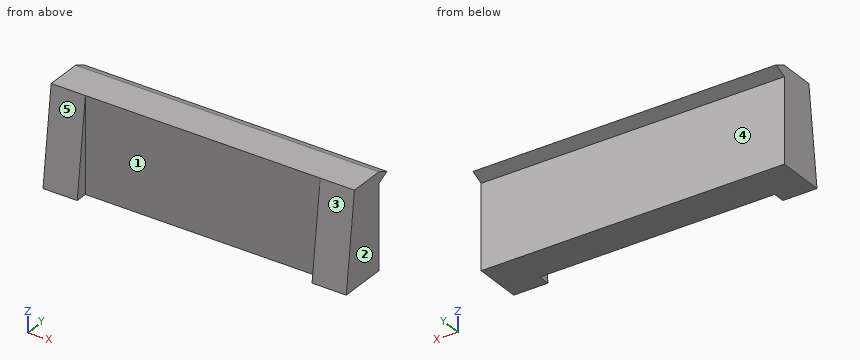
from build123d import *

# Parameters (mm, degrees)
F1_DEPTH = 12.75
F2_W     = 9.87
F2_H     = 0.5
F3_DEPTH = 4.001


with BuildPart() as f1:
    # F0 (on Right) → F1 (new body)
    with BuildSketch(Plane.YZ):
        Polygon((1.5, 4), (0, 4), (-0.5, 0), (1.5, 0), (1.5, 3.533692), (2, 3.766846), align=None)
    extrude(amount=F1_DEPTH)

    # F2 (on face) → F3 (cut, through all)
    with BuildSketch(Plane(origin=(0, 0, 0), x_dir=(1, 0, 0), z_dir=(0, 0, -1))):
        with Locations((6.375, 0.25)):
            Rectangle(F2_W, F2_H)
    extrude(amount=-F3_DEPTH, mode=Mode.SUBTRACT)


solid = f1.part
Here's how the part is built. I have some questions about the finished solid (model axes, mm). Face numbers are marked on the shaded views. A direction names the side the tool comes from. Coordinates: 2 decimals unless noted, no trailing zeros. Order: outer loops, then holes, each group sorted by start corner. A loop starts at its lowest first (then second) coordinate and runs counter-clockwise, first axis right, second up.
Item 1: If we mould it in two halves opening along X, with no side actions, what happens to the marked faces 1, 2 and 3? For each: +X half, -X half, draft (parallel to the pull), parting line (faces both ways), or undercut.
Result sheet:
face 1: undercut
face 2: +X half
face 3: draft
Item 2: I need wall thicknesses on line 1 (Y direction, x = 6, z = 1.05); line 2 (Z direction, x = 9, y = 1.55); line 3 (Y direction, x = 12, z = 2.75). Which ranges of each line are inside material? Lowest first, please.
Result sheet:
line 1: y = 0 to 1.5
line 2: z = 3.56 to 3.98
line 3: y = -0.16 to 1.5
Item 3: For P1, Ø1.8, axis at x = 8, z = 1.5, coming from the +Y side; P2, Ø1.5, axis at x = 11, z = 3.5, coming from the +Y side, each with a flat end and sliding along its axis, tell me the tip position at first contact or that it passes through.
Result sheet:
P1: stops at y = 1.5
P2: stops at y = 2
Item 4: For the marked faces 4 and 5, which set-ups out of +Z, -Z, +X, -X, +Y, -Y let a thin tool reach every point of the face, with its end or its side?
Result sheet:
face 4: -Z, +X, -X, +Y
face 5: +Z, +X, -X, -Y
Item 5: If we section it at C-C on z = 2.35: List the corners of the cut face in (x, y) for me.
Result sheet:
outline: (0, -0.21) - (1.44, -0.21) - (1.44, 0) - (11.31, 0) - (11.31, -0.21) - (12.75, -0.21) - (12.75, 1.5) - (0, 1.5) - close
Item 6: If we section it at B-B on x = 7.75: List the corners of the cut face in (y, z) for me.
Result sheet:
outline: (0, 0) - (1.5, 0) - (1.5, 3.53) - (2, 3.77) - (1.5, 4) - (0, 4) - close
Item 7: If we section it at A-A on z = 0.8: List the corners of the cut face in (x, y) for me, plus the area to 3 significant figures.
Result sheet:
outline: (0, -0.4) - (1.44, -0.4) - (1.44, 0) - (11.31, 0) - (11.31, -0.4) - (12.75, -0.4) - (12.75, 1.5) - (0, 1.5) - close
area: 20.3 mm2
